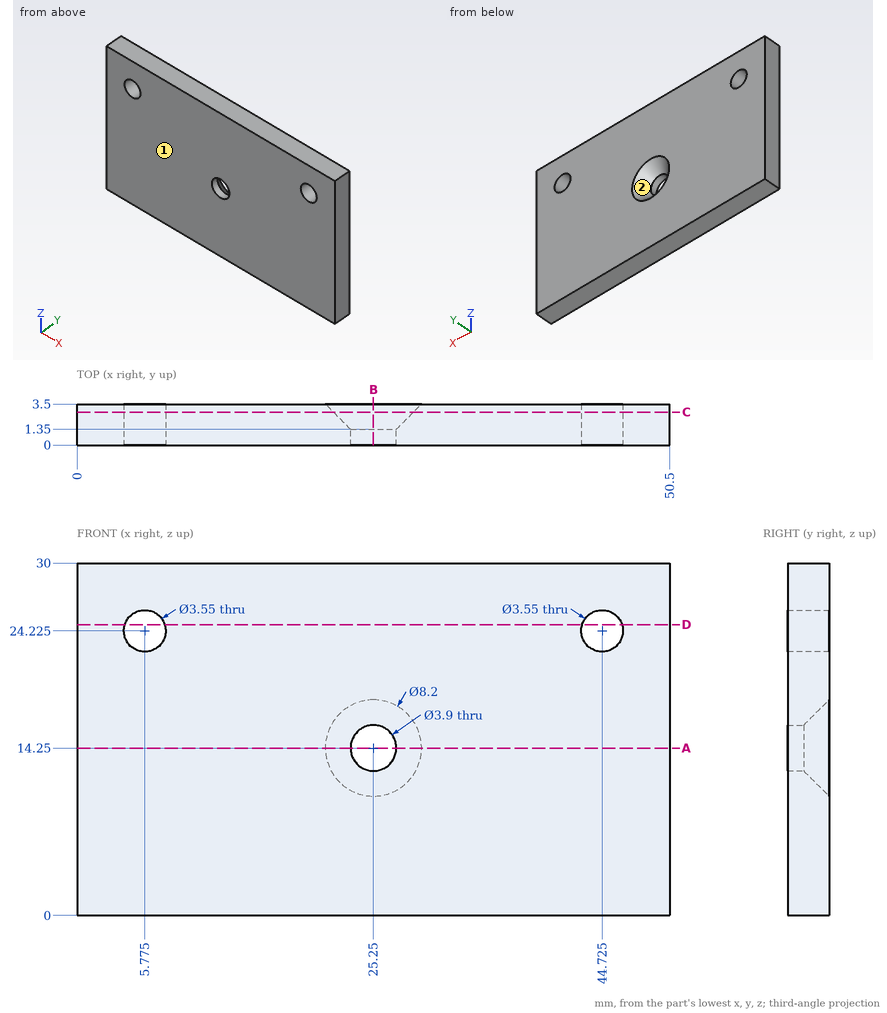
Check sheet for the drawn part. Datum: minimum x, y, z corner. Units: mm. Round coordinates to 2 decimals unless told otherwise and drop trailing zeros. Order: outer loops, then holes, each group sorted by start corner. A loop starts at its lowest first (then second) coordinate and runs counter-clockwise, first axis right, second up. Notation, with made-up numbers: M 10,52.5 L 17,52.5 A31 cw 17,80.5 Z; hole C -1.5,-33 d9. An arc over 180 degrees is marked long. Answer in a Markdown table with one row per item.
(1) Section check C-C on y = 2.8. Record the boundary of the cut face in (x, z) (3 decimals), plus the area to 3 significant figures.
Findings:
| item | result |
|---|---|
| outline | M 0,0 L 50.5,0 L 50.5,30 L 0,30 Z; hole C 5.775,24.225 d3.55; hole C 25.25,14.25 d6.8; hole C 44.725,24.225 d3.55 |
| area | 1,460 mm^2 |
(2) Section check D-D on z = 24.75. Record the boundary of the cut face in (x, y).
Findings:
| item | result |
|---|---|
| outline | M 0,0 L 4.08,0 L 4.08,3.5 L 0,3.5 Z; M 7.47,0 L 43.03,0 L 43.03,3.5 L 7.47,3.5 Z; M 46.42,0 L 50.5,0 L 50.5,3.5 L 46.42,3.5 Z |
(3) Gauge pin test, flat end, axial feed: pin 1 (3 mm diameter, centred on x = 18, z = 10.5, fed in from -Y). Record the tip position at first contact, or that the pin passes through.
Findings:
| item | result |
|---|---|
| pin 1 | stops at y = 0 |
(4) Section check B-B on x = 25.25. Record the boundary of the cut face in (y, z), plus the area to 3 significant figures.
Findings:
| item | result |
|---|---|
| outline | M 0,0 L 3.5,0 L 3.5,10.15 L 1.35,12.3 L 0,12.3 Z; M 0,16.2 L 1.35,16.2 L 3.5,18.35 L 3.5,30 L 0,30 Z |
| area | 86.7 mm^2 |
(5) Section check A-A on z = 14.25. Record the boundary of the cut face in (x, y), plus the area to 3 significant figures.
Findings:
| item | result |
|---|---|
| outline | M 0,0 L 23.3,0 L 23.3,1.35 L 21.15,3.5 L 0,3.5 Z; M 27.2,0 L 50.5,0 L 50.5,3.5 L 29.35,3.5 L 27.2,1.35 Z |
| area | 158 mm^2 |
(6) Draft check along Z on the marked faces 1 and 2. Enter one of: +Z half, -Z half, draft (parallel to the pull), parting line (faces both ways), or undercut.
Findings:
| item | result |
|---|---|
| face 1 | draft |
| face 2 | undercut |
(7) Material ranges on line 1 along Z through (x, y) = (25.25, 1); line 2 along X through (y, z) = (2.65, 23.75); line 3 along X through (y, z) = (0.7, 25.25), recorded low to high. Write a range as from..to.
Findings:
| item | result |
|---|---|
| line 1 | z = 0..12.3, 16.2..30 |
| line 2 | x = 0..4.06, 7.49..43.01, 46.44..50.5 |
| line 3 | x = 0..4.33, 7.22..43.28, 46.17..50.5 |
